Autodesk Inventor part; units mm, degrees
ref_plane "YZ Plane" through (0, 0, 0) normal (1, 0, 0) x (0, 1, 0)
ref_plane "XZ Plane" through (0, 0, 0) normal (0, 1, 0) x (-1, 0, 0)
ref_plane "XY Plane" through (0, 0, 0) normal (0, 0, 1) x (1, 0, 0)
sketch "Sketch1" plane through (0, 0, 0) normal (0, 0, 1) x (1, 0, 0)
  line L0 (-6.5, 0) -> (6.5, 0)
  line L1 (6.5, 0) -> (6.5, 7)
  line L2 (6.5, 7) -> (-6.5, 7)
  line L3 (-6.5, 7) -> (-6.5, 0)
  point P0 (0, 0)
  point P1 (0, 0)
  dimension "d0" = 13
  dimension "d1" = 7
extrude "Extrusion1" add sketch "Sketch1" along normal blind 6.5
sketch "Sketch2" plane through (0, 0, 0) normal (0, 0, -1) x (-1, 0, 0)
  line L0 (-3, 5.5) -> (3, 5.5)
  line L1 (3, 5.5) -> (3, 1.5)
  line L2 (3, 1.5) -> (-3, 1.5)
  line L3 (-3, 1.5) -> (-3, 5.5)
  line L4 (6.5, 0) -> (-6.5, 0)
  line L5 (-6.5, 0) -> (-6.5, 7)
  point P0 (0, 0)
  point P1 (0, 1.5)
  point P2 (0, 0)
  point P3 (-3, 3.5)
  point P4 (-6.5, 3.5)
  dimension "d4" = 4
  dimension "d5" = 6
extrude "Extrusion2" cut sketch "Sketch2" against normal blind 0.1
sketch "Sketch3" plane through (0, 0, 0.1) normal (0, 0, -1) x (-1, 0, 0)
  line L0 (-3, 1.5) -> (-3, 5.5)
  line L1 (3, 1.5) -> (-3, 1.5)
  line L2 (-3, 5.5) -> (0, 5.5)
  line L3 (0, 5.5) -> (0, 1.5)
  line L4 (0, 1.5) -> (-3, 1.5)
  line L5 (-3, 1.5) -> (-3, 5.5)
  point P0 (0, 0)
extrude "Extrusion3" add sketch "Sketch3" along normal blind 5
sketch "Sketch4" plane through (0, 0, 0) normal (1, 0, 0) x (0, 1, 0)
  line L0 (0, 6.5) -> (7, 6.5)
  line L1 (4, 6.5) -> (4, 11.5)
  line L2 (4, 11.5) -> (-2, 11.5)
  line L3 (-2, 11.5) -> (-2, 10.5)
  line L4 (-2, 10.5) -> (3, 10.5)
  line L5 (3, 10.5) -> (3, 6.5)
  line L6 (3, 9) -> (2.5, 8.1738)
  line L7 (2.5, 8.1738) -> (2.5, 6.5)
  line L8 (4, 9) -> (4.5, 8.1738)
  line L9 (4.5, 8.1738) -> (4.5, 6.5)
  line L10 (0, 0) -> (0, 6.5)
  line L11 (4, 9) -> (3, 9) construction
  point P0 (-2, 11)
  point P1 (3.5, 9)
  point P2 (3.5, 6.5)
  dimension "d10" = 1
  dimension "d11" = 1
  dimension "d12" = 2
  dimension "d13" = 2
  dimension "d14" = 5
extrude "Extrusion4" add sketch "Sketch4" along normal mid plane 0.5
pattern_linear "Rectangular Pattern1" count 2 spacing 5 along (-1, 0, 0) of "Extrusion4"
mirror "Mirror1" about plane through (0, 0, 0) normal (1, 0, 0) of "Extrusion4", "Rectangular Pattern1"
properties part number "Switch"
Geometry check sheet. Reference: the model listing, model coordinates, mm. A direction names the side the tool comes from. Give positions to 0.01 mm unless a question says otherwise; leave off trailing zeros. Order: outer loops, then holes, each group sorted by start corner. A loop starts at its lowest first (then second) coordinate and runs counter-clockwise, first axis right, second up.
1. Thickness scan on L1, parallel to Z at x = -0.75, y = 5.75; L2, parallel to Y at x = -5, z = 0.5; L3, parallel to X at y = 2, z = -3.75. Record the ranges inside material, lowest first.
2. Section check D-D, the plane y = 2. Enter the section's corners in (x, z), and give its area (3 significant figures).
3. Access from +Z, -Z, +X, -X, +Y, -Y to the whole of each face (thin tool, end or side, straight path). Record for faces 1 (the face through (-5.25, 2, 11)), 2 (the face through (1, 1.5, -2)), 3 (the face through (3, 3, -2)).
4. Section check A-A, the plane y = 0.75. Enter the section's corners in (x, z).
5. Release check for a two-part mould opening along Y. For faces 4 (the face through (2, 5.5, -2)), 5 (the face through (-6.5, 4, 3)), 6 (the face through (-1, 4, 0.1)) record: pulls with the +Y half, pulls with the -Y half, needs draft (parallel to the pull), parting line crosses it, or undercut.
6. Gauge pin test, flat ends, axial feed: pin 1 Ø1.2 at (y, z) = (2.5, -2.5) entering from +X; pin 2 Ø1 at (x, y) = (-4.5, 3.5) entering from +Z; pin 3 Ø3 at (x, z) = (-1, 3) entering from -Y; pin 4 Ø0.6 at (x, z) = (-5, 7.5) entering from -Y. Record the tip position at first contact, or that the pin passes through.
7. Section check B-B, the plane z = 9.25. Enter the section's corners in (x, y).
8. Section check C-C, the plane x = 5. Enter the section's corners in (y, z), and give its area (3 significant figures).
Values follow:
1. L1: z = 0 to 6.5
1. L2: y = 0 to 7
1. L3: x = 0 to 3
2. outline: (-6.5, 0) - (-3, 0) - (-3, 0.1) - (0, 0.1) - (0, -4.9) - (3, -4.9) - (3, 0) - (6.5, 0) - (6.5, 6.5) - (-6.5, 6.5) - close; (-5.25, 10.5) - (-4.75, 10.5) - (-4.75, 11.5) - (-5.25, 11.5) - close; (-0.25, 10.5) - (0.25, 10.5) - (0.25, 11.5) - (-0.25, 11.5) - close; (4.75, 10.5) - (5.25, 10.5) - (5.25, 11.5) - (4.75, 11.5) - close
2. area: 100 mm2
3. face 1: +Z, -X, +Y, -Y
3. face 2: -Z, +X, -X, -Y
3. face 3: -Z, +X, +Y, -Y
4. outline: (-6.5, 0) - (6.5, 0) - (6.5, 6.5) - (-6.5, 6.5) - close; (-5.25, 10.5) - (-4.75, 10.5) - (-4.75, 11.5) - (-5.25, 11.5) - close; (-0.25, 10.5) - (0.25, 10.5) - (0.25, 11.5) - (-0.25, 11.5) - close; (4.75, 10.5) - (5.25, 10.5) - (5.25, 11.5) - (4.75, 11.5) - close
5. face 4: pulls with the +Y half
5. face 5: needs draft
5. face 6: undercut
6. pin 1: stops at x = 3
6. pin 2: stops at z = 11.5
6. pin 3: stops at y = 0
6. pin 4: stops at y = 2.5
7. outline: (-5.25, 3) - (-4.75, 3) - (-4.75, 4) - (-5.25, 4) - close; (-0.25, 3) - (0.25, 3) - (0.25, 4) - (-0.25, 4) - close; (4.75, 3) - (5.25, 3) - (5.25, 4) - (4.75, 4) - close
8. outline: (-2, 10.5) - (3, 10.5) - (3, 9) - (2.5, 8.17) - (2.5, 6.5) - (0, 6.5) - (0, 0) - (7, 0) - (7, 6.5) - (4.5, 6.5) - (4.5, 8.17) - (4, 9) - (4, 11.5) - (-2, 11.5) - close
8. area: 57.6 mm2
